```python
from build123d import *

# Parameters (mm, degrees)
EXTRUDE_1_DEPTH     = 2
SKETCH_2_R          = 1.65
CUT_EXTRUDE_1_DEPTH = 2
SKETCH_3_R          = 1.75
SKETCH_3_R_2        = 13
CUT_EXTRUDE_2_DEPTH = 2
SKETCH_4_W          = 15
SKETCH_4_H          = 22.74802609
CUT_EXTRUDE_3_DEPTH = 5


with BuildPart() as part:
    # 草图1 → 凸台-拉伸1 (new body)
    with BuildSketch(Plane.XY):
        with BuildLine():
            Line((-43.802574587, 23.289899283), (-34.080892972, 50))
            Line((-34.080892972, 50), (34.080892972, 50))
            Line((34.080892972, 50), (43.802574587, 23.289899283))
            ThreePointArc((43.802574587, 23.289899283), (45.633155509, 20.904239779), (48.501037691, 20))
            Line((48.501037691, 20), (65, 20))
            Line((65, 20), (65, -20))
            Line((65, -20), (-65, -20))
            Line((-65, -20), (-65, 20))
            Line((-65, 20), (-48.501037691, 20))
            ThreePointArc((-48.501037691, 20), (-45.633155509, 20.904239779), (-43.802574587, 23.289899283))
        make_face()
    extrude(amount=EXTRUDE_1_DEPTH)

    # 草图2 → 切除-拉伸1 (cut)
    with BuildSketch(Plane.XY):
        with Locations((-55, -10)):
            Circle(SKETCH_2_R)
        with Locations(Location((55, -10, 0), (0, 0, 180))):
            Circle(SKETCH_2_R)
    extrude(amount=CUT_EXTRUDE_1_DEPTH, mode=Mode.SUBTRACT)

    # 草图3 → 切除-拉伸2 (cut)
    with BuildSketch(Plane.XY):
        with Locations((0, 38)):
            Circle(SKETCH_3_R)
        with Locations((17, 21)):
            Circle(SKETCH_3_R)
        with Locations((0, 4)):
            Circle(SKETCH_3_R)
        with Locations((-17, 21)):
            Circle(SKETCH_3_R)
        with Locations((0, 21)):
            Circle(SKETCH_3_R_2)
    extrude(amount=CUT_EXTRUDE_2_DEPTH, mode=Mode.SUBTRACT)

    # 草图4 → 切除-拉伸3 (cut, symmetric)
    with BuildSketch(Plane.XY.offset(2)):
        with Locations((0, 38.625986955)):
            Rectangle(SKETCH_4_W, SKETCH_4_H)
    extrude(amount=CUT_EXTRUDE_3_DEPTH, both=True, mode=Mode.SUBTRACT)


solid = part.part
```
Input: part model. Units: mm. Frame: model coordinates. Round coordinates to 2 decimals unless told otherwise and drop trailing zeros. Loops run counter-clockwise (first coordinate to the right, second up) from the corner with the lowest first, then second, coordinate; pieces in that order, holes last.
1) Section query C-C on z = 0.4. Return the cut outline in (x, y), plus the area to 3 significant figures.
Ans:
outline: (-65, -20) - (65, -20) - (65, 20) - (48.5, 20) arc R5 cw to (43.8, 23.29) - (34.08, 50) - (7.5, 50) - (7.5, 31.62) arc R13 cw (long way) to (-7.5, 31.62) - (-7.5, 50) - (-34.08, 50) - (-43.8, 23.29) arc R5 cw to (-48.5, 20) - (-65, 20) - close; hole circle Ø3.3 at (-55, -10); hole circle Ø3.5 at (-17, 21); hole circle Ø3.5 at (0, 4); hole circle Ø3.5 at (17, 21); hole circle Ø3.3 at (55, -10)
area: 6,750 mm2
2) Pull-direction query (Y, two-part tool) for faces 1 (the cylindrical face through (-17.228, 22.735, 0.986)), 2 (the flat face through (-39.01, 36.46, 0.99)), 3 (the flat face through (0.9, 7.7, 2)); classes: released by +Y, released by -Y, zero draft, split by the parting line, or undercut.
Ans:
face 1: undercut
face 2: released by +Y
face 3: zero draft
3) Section query D-D on y = 4. Return the cut outline in (x, z).
Ans:
outline: (-65, 0) - (-1.75, 0) - (-1.75, 2) - (-65, 2) - close; (1.75, 0) - (65, 0) - (65, 2) - (1.75, 2) - close
4) Section query A-A on y = -10. Return the cut outline in (x, z).
Ans:
outline: (-65, 0) - (-56.65, 0) - (-56.65, 2) - (-65, 2) - close; (-53.35, 0) - (53.35, 0) - (53.35, 2) - (-53.35, 2) - close; (56.65, 0) - (65, 0) - (65, 2) - (56.65, 2) - close
5) Material intervals for line 1 (Y direction, x = -17, z = 1.4); line 2 (Y direction, x = 0, z = 1.2); line 3 (X direction, y = -8.5, z = 1.2), sorted ascending.
Ans:
line 1: y = -20 to 19.25, 22.75 to 50
line 2: y = -20 to 2.25, 5.75 to 8
line 3: x = -65 to -55.69, -54.31 to 54.31, 55.69 to 65
6) Section query B-B on x = 55. Return the cut outline in (y, z), plus the area to 3 significant figures.
Ans:
outline: (-20, 0) - (-11.65, 0) - (-11.65, 2) - (-20, 2) - close; (-8.35, 0) - (20, 0) - (20, 2) - (-8.35, 2) - close
area: 73.4 mm2
7) Pin query (flat end, axial travel): pin 1 (1 mm diameter, centred on x = -59, z = 1, fed in from +Y). Return the tip coordinate at first contact, or that it passes through.
Ans:
pin 1: stops at y = 20
